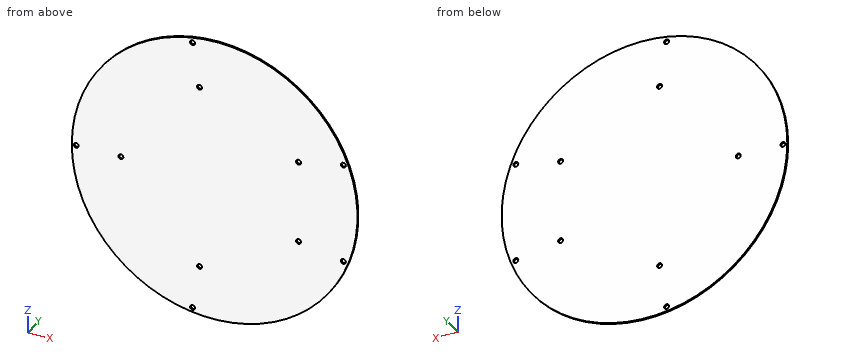
Autodesk Inventor part; units mm, degrees
ref_plane "YZ Plane" through (0, 0, 0) normal (1, 0, 0) x (0, 1, 0)
ref_plane "XZ Plane" through (0, 0, 0) normal (0, 1, 0) x (-1, 0, 0)
ref_plane "XY Plane" through (0, 0, 0) normal (0, 0, 1) x (1, 0, 0)
sketch "Sketch1" plane through (0, 0, 0) normal (0, 1, 0) x (-1, 0, 0)
  circle A0 centre (-2.1062, 1.0257) radius 576.435
  circle A1 centre (-340.5404, 165.8456) radius 10
  circle A2 centre (-521.3675, 200.9948) radius 10
  line L0 (-296.1915, 1.3356) -> (-698.7298, 1.3356)
  circle A3 centre (-340.5404, -163.1743) radius 10
  circle A4 centre (-521.3675, -198.3235) radius 10
  circle A5 centre (376.435, 0) radius 10
  circle A6 centre (556.435, 0) radius 10
  circle A7 centre (58.8874, 371.8005) radius 10
  circle A8 centre (87.0456, 549.5844) radius 10
  circle A9 centre (58.8874, -371.8005) radius 10
  circle A10 centre (87.0456, -549.5844) radius 10
  point P0 (0, 0)
  point P1 (-578.5411, 1.3356)
  dimension "d34" = 1152.87
  dimension "d52" = 20
  dimension "d55" = 20
  dimension "d58" = 556.435
  dimension "d59" = 20
  dimension "d60" = 376.435
  dimension "d61" = 20
  dimension "d62" = 556.435
  dimension "d65" = 81
  dimension "d69" = 81
extrude "Extrusion1" add sketch "Sketch1" along normal blind 7
properties part number "TopandBase"
Could you check a few things on this model? Use its own coordinates, in mm. Give positions to 0.01 mm unless a question says otherwise; leave off trailing zeros. Write each loop counter-clockwise with the first axis right and the second up, starting at its lowest first coordinate (ties: lowest second). Pieces come first, ordered by that corner, then holes. Notation, with made-up numbers: (44.25, 37) - (82.25, 37) arc R25 cw to (82.25, 68) - close; hole circle Ø1 at (45.25, 34.5). An arc over 180 degrees is marked (long way). Use CSV: the item, a comma, the result in double quotes. Start each with the question number.
Item 1: I want a section at B-B, the plane x = 412.5. Please give me the cut outline in (y, z).
Item 2: I'm going to push flat-ended pins straight in: pin 1 (2 mm diameter, centred on x = 12, y = 2, fed in from -Z); pin 2 (1.5 mm diameter, centred on y = 5, z = -443, fed in from -X); pin 3 (1 mm diameter, centred on y = 3.5, z = -205, fed in from +X). Where does each tip first touch, or does it pass through?
Item 3: I want a section at C-C, the plane z = 279. Please give me the cut outline in (x, y).
Item 4: If I drill on line 1 along X through (y, z) = (1, -16); line 2 along X through (y, z) = (5.75, 172.5); line 3 along X through (y, z) = (3.75, -375), over which ranges is the centre line in solid material (lowest first)?
Item 5: I want a section at A-A, the plane y = 5.75. Give the number of separate pieces and of enclosed holes in the cut face, then the cut area to 3 significant figures.
Findings:
1,outline,"(0, -403.76) - (7, -403.76) - (7, 405.81) - (0, 405.81) - close"
2,pin 1,"stops at z = -575.34"
2,pin 2,"stops at x = -366.38"
2,pin 3,"stops at x = 540.66"
3,outline,"(-502.88, 0) - (507.09, 0) - (507.09, 7) - (-502.88, 7) - close"
4,line 1,"x = -574.08 to 578.29"
4,line 2,"x = -548.23 to 333.08, 348 to 552.45"
4,line 3,"x = -434.79 to -68.36, -49.41 to 439.01"
5,separate pieces,"1"
5,enclosed holes,"10"
5,area,"1,040,000 mm2"
